Part print with two shaded views. Sizes in mm from the minimum x, y, z corner. Coordinates: 2 decimals unless noted, no trailing zeros. Loops run counter-clockwise (first coordinate to the right, second up) from the corner with the lowest first, then second, coordinate; pieces in that order, holes last. Notation, with made-up numbers: (-3, -3.75) -> (6, -3.75) arc R20 ccw to (6, 6.25) -> close; hole circle Ø4 at (-28, -8). An arc over 180 degrees is marked (long way). Write each question's results on one line, items separated by ' | '.
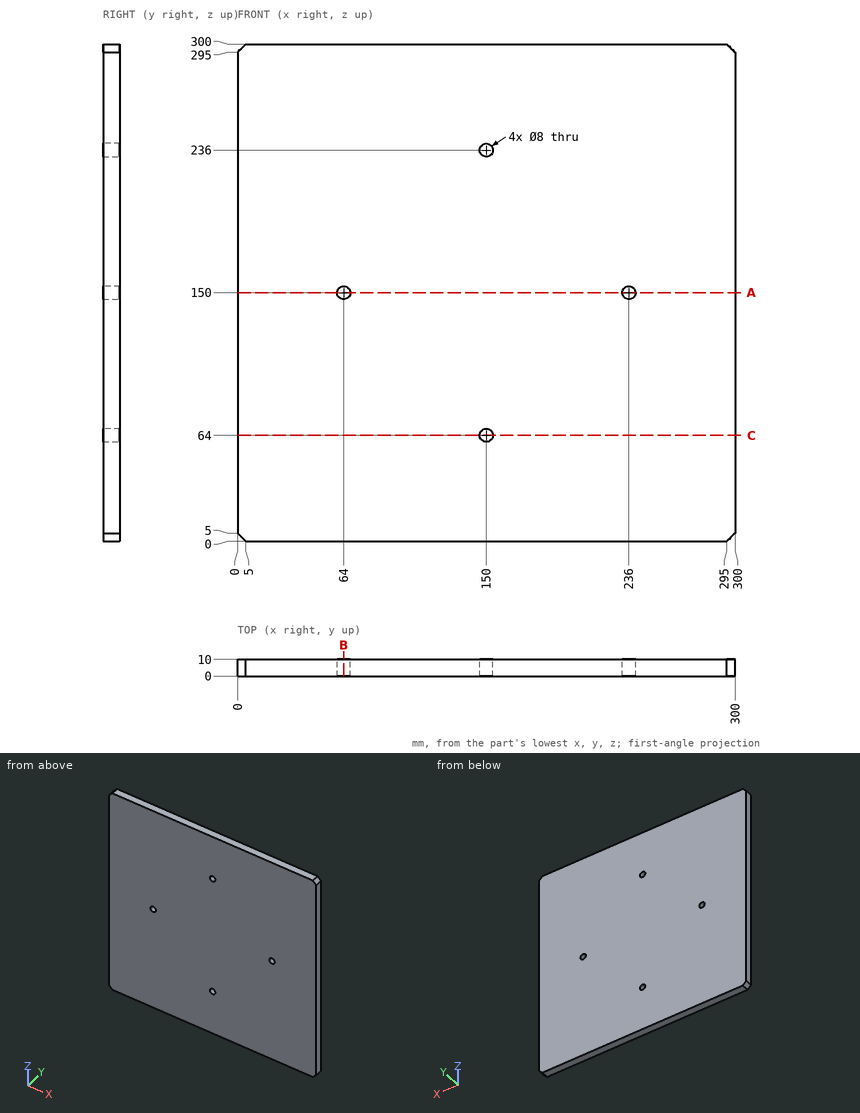
Q1. Wall check: L1, parallel to X at y = 6, z = 150; L2, parallel to X at y = 6.25, z = 64; L3, parallel to X at y = 8, z = 67. Give the ranges that are in metal, low to high. Write a range as from..to.
Results are:
L1: 0..60, 68..232, 240..300 | L2: 0..146, 154..300 | L3: 0..147.35, 152.65..300
Q2. Cut at C-C on z = 64. Write the cut outline in (x, y).
Results are:
outline: (0, 0) -> (146, 0) -> (146, 10) -> (0, 10) -> close; (154, 0) -> (300, 0) -> (300, 10) -> (154, 10) -> close
Q3. Drop a flat-ended pin along its axis: pin 1 (5 mm diameter, centred on x = 236, z = 150, fed in from -Y). Give the stop position or say it passes through.
Results are:
pin 1: through
Q4. Cut at A-A on z = 150. Write the cut outline in (x, y).
Results are:
outline: (0, 0) -> (60, 0) -> (60, 10) -> (0, 10) -> close; (68, 0) -> (232, 0) -> (232, 10) -> (68, 10) -> close; (240, 0) -> (300, 0) -> (300, 10) -> (240, 10) -> close
Q5. Cut at B-B on x = 64. Write the cut outline in (y, z).
Results are:
outline: (0, 0) -> (10, 0) -> (10, 146) -> (0, 146) -> close; (0, 154) -> (10, 154) -> (10, 300) -> (0, 300) -> close
